Could you check a few things on this model? Use its own coordinates, in mm. Face numbers are marked on the shaded views. A direction names the side the tool comes from. Round coordinates to 2 decimals unless told otherwise and drop trailing zeros. Loops run counter-clockwise (first coordinate to the right, second up) from the corner with the lowest first, then second, coordinate; pieces in that order, holes last. Notation, with made-up numbers: (39, -35.75) - (60, -35.75) arc R7 cw to (60, -22.75) - close; hole circle Ø5 at (-23, 42.25). An arc over 180 degrees is marked (long way). Answer as CSV lines item,"result". Start each with the question number.
1) Suppose I cut it at D-D, the plane x = 30. Write out the boundary of the cut face in (y, z), then the cut area to 3 significant figures.
2) We'd pull the mould along X, two halves only. Please class the marked faces 1, 2 and 3: pulls with the +X half, pulls with the -X half, needs draft (parallel to the pull), parting line crosses it, or undercut.
3) I'm going to push a flat-ended pin straight in: pin 1 Ø6 at (x, y) = (52, 7.125) entering from -Z. Where does the tip first touch, or does it pass through?
4) Suppose I cut it at C-C, the plane y = -22. Write out the boundary of the cut face in (x, z).
5) Suppose I cut it at A-A, the plane x = 52. Write out the boundary of the cut face in (y, z) (3 decimals).
6) Please list where these lines run through material, in increasing order: line 1 along Y through (x, z) = (52, 7.25) (3 decimals); line 2 along Y through (x, z) = (10.25, 5.25) (3 decimals); line 3 along X through (y, z) = (-43.5, 12.75).
7) Which directions (+Z, -Z, +X, -X, +Y, -Y) give clear straight access to the entire face, cutting with the end or side of a thin tool? Please do the marked faces 4 and 5.
8) Suppose I cut it at B-B, the plane z = 3. Count the separate pieces of the cut face and the enclosed holes in it, then the cut area to 3 significant figures.
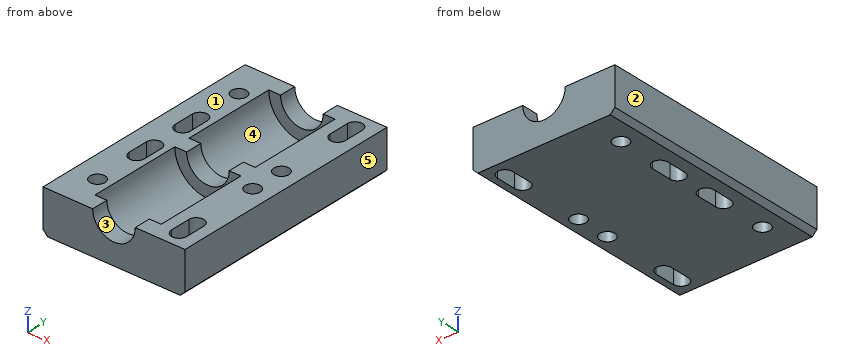
Autodesk Inventor part; units mm, degrees
ref_plane "YZ Plane" through (0, 0, 0) normal (1, 0, 0) x (0, 1, 0)
ref_plane "XZ Plane" through (0, 0, 0) normal (0, 1, 0) x (-1, 0, 0)
ref_plane "XY Plane" through (0, 0, 0) normal (0, 0, 1) x (1, 0, 0)
sketch "Sketch1" plane through (0, 0, 0) normal (0, 0, 1) x (1, 0, 0)
  line L0 (-60, 50) -> (60, 50)
  line L1 (60, 50) -> (60, -50)
  line L2 (60, -50) -> (-60, -50)
  line L3 (-60, -50) -> (-60, 50)
  point P0 (0, 0)
  point P1 (-60, 0)
  point P2 (0, 50)
  dimension "d0" = 120
  dimension "d1" = 100
extrude "Extrusion1" add sketch "Sketch1" along normal blind 18
sketch "Sketch2" plane through (-60, 50, 0) normal (0, 1, 0) x (1, 0, 0)
  line L0 (0, 0) -> (120, 0)
  line L1 (0, 0) -> (0, -18)
  line L2 (120, -18) -> (0, -18)
  line L3 (120, 0) -> (120, -18)
  line L4 (120, -18) -> (0, -18)
  circle A0 centre (30, -18) radius 14
  circle A1 centre (90, -18) radius 14
  circle A2 centre (60, -18) radius 4.5
  point P0 (60, 0)
  dimension "d4" = 28
  dimension "d5" = 9
  dimension "d11" = 30
  dimension "d12" = 30
extrude "Extrusion2" cut sketch "Sketch2" against normal through all contours A0 L2 | L2 A0 | A1 L2 | L2 A1 | A2 L2 | L2 A2
sketch "Sketch3" plane through (0, 0, 18) normal (0, 0, 1) x (1, 0, 0)
  line L0 (16, -50) -> (16, 50)
  line L1 (16, 50) -> (4.5, 50)
  line L2 (4.5, 50) -> (4.5, -50)
  line L3 (4.5, -50) -> (16, -50)
  line L4 (-4.5, -50) -> (-4.5, 50)
  line L5 (-4.5, 50) -> (-16, 50)
  line L6 (-16, 50) -> (-16, -50)
  line L7 (-16, -50) -> (-4.5, -50)
  line L8 (-44, -50) -> (-44, 50)
  line L9 (-44, 50) -> (-60, 50)
  line L10 (-60, 50) -> (-60, -50)
  line L11 (-60, -50) -> (-44, -50)
  line L12 (44, 50) -> (44, -50)
  line L13 (44, -50) -> (60, -50)
  line L14 (60, -50) -> (60, 50)
  line L15 (60, 50) -> (44, 50)
  line L16 (-60, 50) -> (60, 50) construction
  line L17 (-52, 50) -> (-52, -50) construction
  line L18 (52, 50) -> (52, -50) construction
  line L19 (16, 50) -> (4.5, 50) construction
  line L20 (10.25, 50) -> (10.25, -50) construction
  line L21 (4.5, -50) -> (16, -50) construction
  line L22 (-10.25, 50) -> (-10.25, -50) construction
  line L23 (-16, -50) -> (-4.5, -50) construction
  circle A0 centre (-52, 35) radius 3.2
  circle A1 centre (-52, -35) radius 3.2
  circle A2 centre (52, 35) radius 3.2
  circle A3 centre (52, -35) radius 3.2
  circle A4 centre (-10.25, 35) radius 3.2
  circle A5 centre (10.25, 35) radius 3.2
  circle A6 centre (-10.25, -35) radius 3.2
  circle A7 centre (10.25, -35) radius 3.2
  dimension "d13" = 15
  dimension "d14" = 15
  dimension "d15" = 6.4
extrude "Extrusion3" cut sketch "Sketch3" against normal through all contours A0 | A1 | A2 | A3 | A4 | A5 | A6 | A7
sketch "Sketch6" plane through (0, 0, 0) normal (0, 0, -1) x (-1, 0, 0)
  circle A0 centre (-52, 35) radius 3.2
  circle A1 centre (52, 35) radius 3.2
  circle A2 centre (10.25, 35) radius 3.2
  circle A3 centre (-10.25, 35) radius 3.2
  circle A4 centre (-10.25, -35) radius 3.2
  circle A5 centre (10.25, -35) radius 3.2
  circle A6 centre (52, -35) radius 3.2
  circle A7 centre (-52, -35) radius 3.2
  line L0 (60, 50) -> (-60, 50)
  line L1 (-60, 50) -> (-60, -50)
  line L2 (-60, -50) -> (60, -50)
  line L3 (60, -50) -> (60, 50)
  line L4 (52, 7.125) -> (-52, 7.125) construction
  line L5 (-52, 7.125) -> (-52, -7.125) construction
  line L6 (-52, -7.125) -> (52, -7.125) construction
  line L7 (52, -7.125) -> (52, 7.125) construction
  circle A8 centre (-52, -7.125) radius 3.2
  circle A9 centre (52, -7.125) radius 3.2
  circle A10 centre (10.25, -7.125) radius 3.2
  circle A11 centre (-10.25, -7.125) radius 3.2
  circle A12 centre (-10.25, 7.125) radius 3.2
  circle A13 centre (10.25, 7.125) radius 3.2
  circle A14 centre (52, 7.125) radius 3.2
  circle A15 centre (-52, 7.125) radius 3.2
  point P0 (0, 0)
  point P1 (0, 7.125)
  point P2 (52, 0)
  dimension "d26" = 14.25
  dimension "d27" = 6.4
extrude "Extrusion6" cut sketch "Sketch6" against normal through all contours A8 | A9 | A10 | A11 | A12 | A13 | A14 | A15
sketch "Sketch7" plane through (0, 0, 0) normal (0, 0, -1) x (-1, 0, 0)
  circle A0 centre (52, 7.125) radius 3.2
  circle A1 centre (-10.25, 7.125) radius 3.2
  circle A2 centre (10.25, -7.125) radius 3.2
  circle A3 centre (-52, -7.125) radius 3.2
  circle A4 centre (52, -7.125) radius 3.2
  circle A5 centre (-10.25, -7.125) radius 3.2
  circle A6 centre (10.25, 7.125) radius 3.2
  circle A7 centre (-52, 7.125) radius 3.2
  circle A8 centre (-52, 35) radius 3.2
  circle A9 centre (52, 35) radius 3.2
  circle A10 centre (10.25, 35) radius 3.2
  circle A11 centre (-10.25, 35) radius 3.2
  circle A12 centre (-10.25, -35) radius 3.2
  circle A13 centre (10.25, -35) radius 3.2
  circle A14 centre (52, -35) radius 3.2
  circle A15 centre (-52, -35) radius 3.2
  line L0 (60, 50) -> (-60, 50)
  line L1 (-60, 50) -> (-60, -50)
  line L2 (-60, -50) -> (60, -50)
  line L3 (60, -50) -> (60, 50)
  line L4 (52, -35) -> (52, -43.5) construction
  line L5 (55.2, -35) -> (55.2, -43.5)
  line L6 (48.8, -43.5) -> (48.8, -35)
  arc A16 (55.2, -35) -> (48.8, -35) centre (52, -35) ccw
  arc A17 (48.8, -43.5) -> (55.2, -43.5) centre (52, -43.5) ccw
  line L7 (-52, -35) -> (-52, -43.5) construction
  line L8 (-55.2, -35) -> (-55.2, -43.5)
  line L9 (-48.8, -43.5) -> (-48.8, -35)
  arc A18 (-48.8, -35) -> (-55.2, -35) centre (-52, -35) ccw
  arc A19 (-55.2, -43.5) -> (-48.8, -43.5) centre (-52, -43.5) ccw
  line L10 (-52, 35) -> (-52, 43.5) construction
  line L11 (-55.2, 35) -> (-55.2, 43.5)
  line L12 (-48.8, 43.5) -> (-48.8, 35)
  arc A20 (-55.2, 35) -> (-48.8, 35) centre (-52, 35) ccw
  arc A21 (-48.8, 43.5) -> (-55.2, 43.5) centre (-52, 43.5) ccw
  line L13 (52, 35) -> (52, 43.5) construction
  line L14 (55.2, 35) -> (55.2, 43.5)
  line L15 (48.8, 43.5) -> (48.8, 35)
  arc A22 (48.8, 35) -> (55.2, 35) centre (52, 35) ccw
  arc A23 (55.2, 43.5) -> (48.8, 43.5) centre (52, 43.5) ccw
  line L16 (10.25, -7.125) -> (10.25, -15.625) construction
  line L17 (13.45, -7.125) -> (13.45, -15.625)
  line L18 (7.05, -15.625) -> (7.05, -7.125)
  arc A24 (13.45, -7.125) -> (7.05, -7.125) centre (10.25, -7.125) ccw
  arc A25 (7.05, -15.625) -> (13.45, -15.625) centre (10.25, -15.625) ccw
  line L19 (-10.25, -7.125) -> (-10.25, -15.625) construction
  line L20 (-7.05, -7.125) -> (-7.05, -15.625)
  line L21 (-13.45, -15.625) -> (-13.45, -7.125)
  arc A26 (-7.05, -7.125) -> (-13.45, -7.125) centre (-10.25, -7.125) ccw
  arc A27 (-13.45, -15.625) -> (-7.05, -15.625) centre (-10.25, -15.625) ccw
  line L22 (-10.25, 7.125) -> (-10.25, 15.625) construction
  line L23 (-7.05, 7.125) -> (-7.05, 15.625)
  line L24 (-13.45, 15.625) -> (-13.45, 7.125)
  arc A28 (-13.45, 7.125) -> (-7.05, 7.125) centre (-10.25, 7.125) ccw
  arc A29 (-7.05, 15.625) -> (-13.45, 15.625) centre (-10.25, 15.625) ccw
  line L25 (10.25, 7.125) -> (10.25, 15.625) construction
  line L26 (13.45, 7.125) -> (13.45, 15.625)
  line L27 (7.05, 15.625) -> (7.05, 7.125)
  arc A30 (7.05, 7.125) -> (13.45, 7.125) centre (10.25, 7.125) ccw
  arc A31 (13.45, 15.625) -> (7.05, 15.625) centre (10.25, 15.625) ccw
  point P0 (0, 0)
  point P1 (52, -39.25)
  point P2 (-52, -39.25)
  point P3 (-52, 39.25)
  point P4 (52, 39.25)
  point P5 (10.25, -11.375)
  point P6 (-10.25, -11.375)
  point P7 (-10.25, 11.375)
  point P8 (10.25, 11.375)
  dimension "d30" = 8.5
  dimension "d31" = 3.2
extrude "Extrusion7" cut sketch "Sketch7" against normal through all contours A1 L24 A29 L23 | L17 A25 L18 A2 | L20 A27 L21 A5 | A6 L27 A31 L26 | A8 L11 A21 L12 | A9 L15 A23 L14 | L5 A17 L6 A14 | L9 A19 L8 A15
sketch "Sketch9" plane through (-60, 50, 0) normal (0, 1, 0) x (1, 0, 0)
  arc A0 (104, -18) -> (76, -18) centre (90, -18) ccw construction
  line L0 (120, -18) -> (104, -18) construction
  line L1 (120, 0) -> (120, -18) construction
  line L2 (0, 0) -> (120, 0) construction
  line L3 (0, 0) -> (0, -18) construction
  line L4 (16, -18) -> (0, -18) construction
  arc A1 (44, -18) -> (16, -18) centre (30, -18) ccw construction
  line L5 (55.5, -18) -> (44, -18) construction
  arc A2 (64.5, -18) -> (55.5, -18) centre (60, -18) ccw
  line L6 (76, -18) -> (64.5, -18) construction
  circle A3 centre (90, -18) radius 8 construction
  circle A4 centre (30, -18) radius 8 construction
  arc A5 (99, -18) -> (81, -18) centre (90, -18) ccw
  arc A6 (39, -18) -> (21, -18) centre (30, -18) ccw
  line L7 (120, -18) -> (104, -18)
  line L8 (21, -18) -> (16, -18)
  line L9 (104, -18) -> (99, -18)
  line L10 (81, -18) -> (76, -18)
  line L11 (44, -18) -> (39, -18)
  arc A7 (104, -18) -> (76, -18) centre (90, -18) ccw
  arc A8 (44, -18) -> (16, -18) centre (30, -18) ccw
  point P0 (60, 0)
  dimension "d37" = 18
extrude "Extrusion9" add sketch "Sketch9" against normal blind 7
ref_plane "Work Plane1" through (-60, 0, 0) normal (0, 1, 0) x (1, 0, 0)
mirror "Mirror1" about plane through (-60, 0, 0) normal (0, 1, 0) of "Extrusion9"
sketch "Sketch10" plane through (-60, 0, 0) normal (0, 1, 0) x (1, 0, 0)
  line L0 (21, -18) -> (16, -18)
  arc A0 (39, -18) -> (21, -18) centre (30, -18) ccw
  line L1 (44, -18) -> (39, -18)
  arc A1 (44, -18) -> (16, -18) centre (30, -18) ccw
  line L2 (104, -18) -> (99, -18)
  arc A2 (104, -18) -> (76, -18) centre (90, -18) ccw
  line L3 (81, -18) -> (76, -18)
  arc A3 (99, -18) -> (81, -18) centre (90, -18) ccw
  point P0 (60, 0)
extrude "Extrusion10" add sketch "Sketch10" along normal mid plane 7
chamfer "Chamfer1" distance 2 angle 45 2 edges at (-60, 0, 0) (60, 0, 0)
sketch "Sketch12" plane through (0, 0, 0) normal (0, 0, -1) x (-1, 0, 0)
  line L0 (-58, -50) -> (-58, 50) construction
  line L1 (-58, -50) -> (58, -50) construction
  line L2 (58, 50) -> (58, -50) construction
  line L3 (58, 50) -> (-58, 50) construction
  line L4 (-48.8, -35) -> (-48.8, -43.5) construction
  arc A0 (-55.2, -43.5) -> (-48.8, -43.5) centre (-52, -43.5) ccw construction
  line L5 (-55.2, -43.5) -> (-55.2, -35) construction
  arc A1 (-48.8, -35) -> (-55.2, -35) centre (-52, -35) ccw construction
  line L6 (55.2, -35) -> (55.2, -43.5) construction
  arc A2 (48.8, -43.5) -> (55.2, -43.5) centre (52, -43.5) ccw construction
  line L7 (48.8, -43.5) -> (48.8, -35) construction
  arc A3 (55.2, -35) -> (48.8, -35) centre (52, -35) ccw construction
  circle A4 centre (10.25, -35) radius 3.2 construction
  circle A5 centre (-10.25, -35) radius 3.2 construction
  circle A6 centre (-10.25, 35) radius 3.2 construction
  circle A7 centre (10.25, 35) radius 3.2 construction
  line L8 (-55.2, 35) -> (-55.2, 43.5) construction
  arc A8 (-48.8, 43.5) -> (-55.2, 43.5) centre (-52, 43.5) ccw construction
  line L9 (-48.8, 43.5) -> (-48.8, 35) construction
  arc A9 (-55.2, 35) -> (-48.8, 35) centre (-52, 35) ccw construction
  circle A10 centre (-52, 7.125) radius 3.2 construction
  line L10 (-7.05, -7.125) -> (-7.05, -15.625) construction
  arc A11 (-13.45, -15.625) -> (-7.05, -15.625) centre (-10.25, -15.625) ccw construction
  line L11 (-13.45, -15.625) -> (-13.45, -7.125) construction
  arc A12 (-7.05, -7.125) -> (-13.45, -7.125) centre (-10.25, -7.125) ccw construction
  circle A13 centre (52, -7.125) radius 3.2 construction
  circle A14 centre (-52, -7.125) radius 3.2 construction
  line L12 (13.45, -7.125) -> (13.45, -15.625) construction
  arc A15 (7.05, -15.625) -> (13.45, -15.625) centre (10.25, -15.625) ccw construction
  line L13 (7.05, -15.625) -> (7.05, -7.125) construction
  arc A16 (13.45, -7.125) -> (7.05, -7.125) centre (10.25, -7.125) ccw construction
  circle A17 centre (52, 7.125) radius 3.2 construction
  line L14 (13.45, 15.625) -> (13.45, 7.125) construction
  arc A18 (7.05, 7.125) -> (13.45, 7.125) centre (10.25, 7.125) ccw construction
  line L15 (7.05, 7.125) -> (7.05, 15.625) construction
  arc A19 (13.45, 15.625) -> (7.05, 15.625) centre (10.25, 15.625) ccw construction
  line L16 (55.2, 43.5) -> (55.2, 35) construction
  arc A20 (48.8, 35) -> (55.2, 35) centre (52, 35) ccw construction
  line L17 (48.8, 35) -> (48.8, 43.5) construction
  arc A21 (55.2, 43.5) -> (48.8, 43.5) centre (52, 43.5) ccw construction
  line L18 (-7.05, 15.625) -> (-7.05, 7.125) construction
  arc A22 (-13.45, 7.125) -> (-7.05, 7.125) centre (-10.25, 7.125) ccw construction
  line L19 (-13.45, 7.125) -> (-13.45, 15.625) construction
  arc A23 (-7.05, 15.625) -> (-13.45, 15.625) centre (-10.25, 15.625) ccw construction
  line L20 (60, 50) -> (58, 50) construction
  line L21 (58, 50) -> (58, -50) construction
  line L22 (58, -50) -> (60, -50) construction
  line L23 (60, -50) -> (60, 50) construction
  line L24 (-60, -50) -> (-58, -50) construction
  line L25 (-58, -50) -> (-58, 50) construction
  line L26 (-58, 50) -> (-60, 50) construction
  line L27 (-60, 50) -> (-60, -50) construction
  line L28 (60, 50) -> (0, 50)
  line L29 (0, 50) -> (0, -50)
  line L30 (0, -50) -> (60, -50)
  line L31 (60, -50) -> (60, 50)
  point P0 (0, 0)
extrude "Extrusion11" cut sketch "Sketch12" against normal through all
sketch "Sketch13" plane through (0, 0, 18) normal (0, 0, 1) x (1, 0, 0)
  line L0 (0, 50) -> (0, -50)
  line L1 (4.5, -50) -> (0, -50)
  line L2 (4.5, 50) -> (4.5, -50)
  line L3 (0, 50) -> (4.5, 50)
  point P0 (0, 0)
extrude "Extrusion12" add sketch "Sketch13" against normal up to surface (18 mm away)
chamfer "Chamfer2" distance 2 angle 45 1 edges at (0, 0, 0)
properties part number "AXCARv4" material "PC/ABS Plastic"
Filled sheet:
1,outline,"(-50, 0) - (50, 0) - (50, 9) - (43, 9) - (43, 4) - (3.5, 4) - (3.5, 9) - (-3.5, 9) - (-3.5, 4) - (-43, 4) - (-43, 9) - (-50, 9) - close"
1,area,"505 mm²"
2,face 1,"needs draft"
2,face 2,"pulls with the -X half"
2,face 3,"undercut"
3,pin 1,"through"
4,outline,"(0, 2) - (2, 0) - (58, 0) - (60, 2) - (60, 18) - (44, 18) arc R14 cw to (16, 18) - (0, 18) - close"
5,outline,"(-50, 0) - (-46.7, 0) - (-46.7, 18) - (-50, 18) - close; (-31.8, 0) - (-10.325, 0) - (-10.325, 18) - (-31.8, 18) - close; (-3.925, 0) - (3.925, 0) - (3.925, 18) - (-3.925, 18) - close; (10.325, 0) - (31.8, 0) - (31.8, 18) - (10.325, 18) - close; (46.7, 0) - (50, 0) - (50, 18) - (46.7, 18) - close"
6,line 1,"-50 to -46.7, -31.8 to -10.325, -3.925 to 3.925, 10.325 to 31.8, 46.7 to 50"
6,line 2,"-50 to -38.2, -31.8 to -18.825, -3.925 to 3.925, 18.825 to 31.8, 38.2 to 50"
6,line 3,"0 to 22.69, 37.31 to 48.8, 55.2 to 60"
7,face 4,"+Z"
7,face 5,"+Z, -Z, +X, +Y, -Y"
8,separate pieces,"1"
8,enclosed holes,"8"
8,area,"5,530 mm²"
